```python
from build123d import *

# Parameters (mm, degrees)
SKETCH1_W           = 27.7
SKETCH1_H           = 15.8
BOSS_EXTRUDE1_DEPTH = 6.3
SKETCH2_OUTSIDE_W   = 36.202
SKETCH2_OUTSIDE_H   = 14.802
CUT_EXTRUDE1_DEPTH  = 15.9
SKETCH3_OUTSIDE_W   = 24.302
SKETCH3_OUTSIDE_H   = 14.802
CUT_EXTRUDE2_DEPTH  = 35.9
BOSS_EXTRUDE2_DEPTH = 6.3
SKETCH5_R           = 2.475
BOSS_EXTRUDE3_DEPTH = 1.9
SKETCH6_W           = 20.8
SKETCH6_H           = 12.8
CUT_EXTRUDE3_DEPTH  = 2


with BuildPart() as part:
    # Sketch1 → Boss-Extrude1 (new body)
    with BuildSketch(Plane(origin=(0, 0, 0), x_dir=(1, 0, 0), z_dir=(0, 1, 0))):
        with Locations((-20.178976781, 7.9)):
            Rectangle(SKETCH1_W, SKETCH1_H)
    extrude(amount=BOSS_EXTRUDE1_DEPTH)

    # Sketch2 outside → Cut-Extrude1 (cut)
    with BuildSketch(Plane.XY):
        with Locations((-20.179, 3.15)):
            Rectangle(SKETCH2_OUTSIDE_W, SKETCH2_OUTSIDE_H)
        with BuildLine():
            Line((-34.028976781, 0), (-10.228976781, 0))
            Line((-10.228976781, 0), (-10.228976781, 1.7))
            add(Edge.make_bspline(
                [(-10.228976781, 1.7), (-9.604071017, 4.446739352), (-6.328976781, 5.206240769)],
                knots=[0, 0, 0, 1, 1, 1], degree=2))
            Line((-6.328976781, 5.206240769), (-6.445984235, 6.3))
            add(Edge.make_bspline(
                [(-14.428976781, 4.3), (-10.215266521, 4.423026161), (-6.445984235, 6.3)],
                knots=[0, 0, 0, 1, 1, 1], degree=2))
            add(Edge.make_bspline(
                [(-26.228976781, 6.3), (-22.205866261, 6.270484551), (-18.300973194, 5.255436261), (-14.428976781, 4.3)],
                knots=[0, 0, 0, 0, 1, 1, 1, 1], degree=3))
            Line((-26.228976781, 6.3), (-34.028976781, 6.3))
            Line((-34.028976781, 6.3), (-34.028976781, 0))
        make_face(mode=Mode.SUBTRACT)
    extrude(amount=-CUT_EXTRUDE1_DEPTH, mode=Mode.SUBTRACT)

    # Sketch3 outside → Cut-Extrude2 (cut)
    with BuildSketch(Plane.ZY.offset(34.028976781)):
        with Locations((-7.9, 3.15)):
            Rectangle(SKETCH3_OUTSIDE_W, SKETCH3_OUTSIDE_H)
        Polygon((-15.8, 0), (-15.8, 3.3), (-12.7, 6.3), (-3.1, 6.3), (0, 3.3), (0, 0), align=None, mode=Mode.SUBTRACT)
    extrude(amount=-CUT_EXTRUDE2_DEPTH, mode=Mode.SUBTRACT)

    # Sketch4 → Boss-Extrude2 (add)
    with BuildSketch(Plane.XZ):
        with BuildLine():
            Line((-34.028976781, -3.9), (-34.028976781, -11.9))
            ThreePointArc((-34.028976781, -11.9), (-30.128976781, -15.8), (-26.228976781, -11.9))
            Line((-26.228976781, -11.9), (-26.228976781, -3.899999628))
            ThreePointArc((-26.228976781, -3.899999628), (-30.128976967, 1.86e-07), (-34.028976781, -3.9))
        make_face()
    extrude(amount=-BOSS_EXTRUDE2_DEPTH)

    # Sketch5 → Boss-Extrude3 (add)
    with BuildSketch(Plane(origin=(0, 6.3, 0), x_dir=(1, 0, 0), z_dir=(0, 1, 0))):
        with Locations(Location((-30.053976781, 11.82570761, 0), (0, 0, 90))):
            Circle(SKETCH5_R)
        with Locations(Location((-30.053976781, 3.974999814, 0), (0, 0, 90))):
            Circle(SKETCH5_R)
    extrude(amount=BOSS_EXTRUDE3_DEPTH)

    # Sketch6 → Cut-Extrude3 (cut)
    with BuildSketch(Plane.XZ):
        with Locations((-22.128976781, -7.9)):
            Rectangle(SKETCH6_W, SKETCH6_H)
    extrude(amount=-CUT_EXTRUDE3_DEPTH, mode=Mode.SUBTRACT)


solid = part.part
```
Model file for the job. Use its own axes, mm. A direction names the side the tool comes from. Coordinates: 2 decimals unless noted, no trailing zeros. Order: outer loops, then holes, each group sorted by start corner. A loop starts at its lowest first (then second) coordinate and runs counter-clockwise, first axis right, second up. Notation, with made-up numbers: (-23, -39.75) -> (14, -39.75) arc R30 ccw to (14, -17.75) -> close; hole circle Ø6 at (70, 13.25). An arc over 180 degrees is marked (long way). Return JSON: item names as keys, results as strings.
Item 1: Slice it at B-B (x = -32.25). Write the cut outline in (y, z), then the cut area to 3 significant figures.
Model answer:
{"outline": "(0, -15.8) -> (3.3, -15.8) -> (3.91, -15.17) -> (6.3, -15.17) -> (6.3, -12.97) -> (8.2, -12.97) -> (8.2, -10.68) -> (6.3, -10.68) -> (6.3, -5.12) -> (8.2, -5.12) -> (8.2, -2.83) -> (6.3, -2.83) -> (6.3, -0.63) -> (3.91, -0.63) -> (3.3, 0) -> (0, 0) -> (0, -1.5) -> (2, -1.5) -> (2, -14.3) -> (0, -14.3) -> close", "area": "79.2 mm²"}
Item 2: Slice it at C-C (y = 7.75). Write the cut outline in (x, z) (3 decimals), then the cut area to 3 significant figures.
Model answer:
{"outline": "circle Ø4.95 at (-30.054, -11.826); circle Ø4.95 at (-30.054, -3.975)", "area": "38.5 mm²"}
Item 3: Mould opens along Z. For faces 1 (the face through (-30.1, 5.1, 0)), 2 (the face through (-22, 2, -8)), 3 (the face through (-11.729, 1, -8)), 4 (the face through (-22, 2, -15.8)) say: pulls with the +Z half, pulls with the -Z half, needs draft (parallel to the pull), parting line crosses it, or undercut.
Model answer:
{"face 1": "pulls with the +Z half", "face 2": "undercut", "face 3": "undercut", "face 4": "pulls with the -Z half"}
Item 4: Slice it at A-A (y = 0.5). Write the cut outline in (x, z).
Model answer:
{"outline": "(-34.03, -15.8) -> (-10.23, -15.8) -> (-10.23, 0) -> (-34.03, 0) -> close; hole (-32.53, -14.3) -> (-11.73, -14.3) -> (-11.73, -1.5) -> (-32.53, -1.5) -> close"}
Item 5: 3-axis set-ups, long thin cutter, end or side, ignore diameter. For faces 5 (the face through (-22, 1, -14.3)), 6 (the face through (-30, 6.3, -8)), 7 (the face through (-18.39, 4.49, -1.23)), 8 (the face through (-18.396, 4.446, -14.616)), 9 (the face through (-33.24, 4.14, -0.87)): which of +Z, -Z, +X, -X, +Y, -Y reach the whole face in a straight line?
Model answer:
{"face 5": "-Y", "face 6": "+Y", "face 7": "+Z, +X, +Y", "face 8": "-Z, +X, +Y", "face 9": "+Z, -X, +Y"}
Item 6: Pin check, flat tips, straight feed: P1, Ø2, axis at x = -23.5, z = -4, coming from the -Y side; P2, Ø3, axis at x = -26, z = -13.5, coming from the -Y side; P3, Ø1.6, axis at y = 1.5, z = -7.5, coming from the +X side; P4, Ø1, axis at x = -16.5, y = 4, coming from the -Z side. Stop position of each tip, or through.
Model answer:
{"P1": "stops at y = 2", "P2": "stops at y = 0", "P3": "stops at x = -10.05", "P4": "stops at z = -15.59"}
Item 7: Wall check: line 1 along X through (y, z) = (0.5, -13.25); line 2 along Z through (x, y) = (-14.5, 1); line 3 along Y through (x, z) = (-28.25, -8.5). Give the ranges that are in metal, low to high. Write a range as from..to.
Model answer:
{"line 1": "x = -34.03..-32.53, -11.73..-10.23", "line 2": "z = -15.8..-14.3, -1.5..0", "line 3": "y = 2..6.3"}
